Verification items for the finished model (mm, model axes). A direction names the side the tool comes from. Round coordinates to 2 decimals unless told otherwise and drop trailing zeros. Write each loop counter-clockwise with the first axis right and the second up, starting at its lowest first coordinate (ties: lowest second). Pieces come first, ordered by that corner, then holes. Notation, with made-up numbers: M 9.25,-17 L 15.25,-17 A16 ccw 15.25,-7 Z; hole C 41.5,-37.75 d7. An arc over 180 degrees is marked long. Answer in a Markdown table with one row per item. Add a question column.
1. Sectioned sample at C-C on z = -5. Record the cut outline in (x, y), plus the area to 3 significant figures.
2. Sectioned sample at D-D on x = 3. Record the cut outline in (y, z).
3. Draft check along Y on faces 1 (the flat face through (5.85, -39.7, -36.85)), 2 (the flat face through (1, -58.005, -16)), 3 (the flat face through (1, -23, -45.183)), 4 (the cylindrical face through (0.78, -37.96, -41.69)). Enter one of: pulls with the +Y half, pulls with the -Y half, needs draft (parallel to the pull), parting line crosses it, or undercut.
4. Go/stop test with flat-tipped pins: pin 1 Ø5 at (y, z) = (-36.61, 10.3) entering from +X; pin 2 Ø2.5 at (y, z) = (3.39, 10.3) entering from -X. Record where each tip stops, or that it passes through.
5. Sectioned sample at A-A on x = 9.5. Record the cut outline in (y, z), plus the area to 3 significant figures.
6. Sectioned sample at B-B on y = -43.5. Record the cut outline in (x, z).
7. Material ranges on probe 1 along X at (y, z) = (-17, -30); probe 2 along Z at (x, y) = (2.5, -43.5); probe 3 along Y at (x, z) = (0.5, 6), recorded low to high.
8. Set-up check for faces 5 (the flat face through (5.85, -45.91, -39.82)), 6 (the flat face through (5.85, -39.7, -40.78)): record each of +Z, -Z, +X, -X, +Y, -Y from which the full face is reachable in a straight line by a thin tool's end or side.
```python
from build123d import *

# Parameters (mm, degrees)
BOSS_EXTRUDE1_DEPTH           = 1.5875
SKETCH2_R                     = 1.524
CUT_EXTRUDE1_DEPTH            = 2.54
SKETCH6_W                     = 2.413
SKETCH6_H                     = 12.7
BOSS_EXTRUDE2_DEPTH           = 8.636
BOSS_EXTRUDE2_DRAFT           = 3
BOSS_EXTRUDE2_PROFILE_2_DEPTH = 8.636
BOSS_EXTRUDE2_PROFILE_2_DRAFT = 3


with BuildPart() as part:
    # Sketch1 → Boss-Extrude1 (new body)
    with BuildSketch(Plane(origin=(0, 0, 0), x_dir=(0, 0, -1), z_dir=(1, 0, 0))):
        with BuildLine():
            Line((45.182706914, 6.18069038), (-13.097593086, 6.18069038))
            Line((-13.097593086, 6.18069038), (-13.097593086, -51.36046962))
            add(Edge.make_bspline(
                [(-13.097593086, -51.36046962), (-13.097593086, -58.00510962), (-0.650340424, -58.00510962)],
                knots=[3.141592654, 3.141592654, 3.141592654, 4.71238898, 4.71238898, 4.71238898], degree=2, weights=[1, 0.707106781, 1]))
            Line((-0.650340424, -58.00510962), (32.623659576, -58.00510962))
            add(Edge.make_bspline(
                [(32.623659576, -58.00510962), (45.182706914, -58.00510962), (45.182706914, -51.36046962)],
                knots=[4.71238898, 4.71238898, 4.71238898, 6.283185307, 6.283185307, 6.283185307], degree=2, weights=[1, 0.707106781, 1]))
            Line((45.182706914, -51.36046962), (45.182706914, -39.42246962))
            Line((45.182706914, -39.42246962), (45.182706914, 6.18069038))
        make_face()
    extrude(amount=BOSS_EXTRUDE1_DEPTH)

    # Sketch2 → Cut-Extrude1 (cut)
    with BuildSketch(Plane.ZY):
        with Locations((-42.388706914, 3.38669038)):
            Circle(SKETCH2_R)
        with Locations((10.303593086, 3.38669038)):
            Circle(SKETCH2_R)
        with Locations((-42.388706914, -36.60560962)):
            Circle(SKETCH2_R)
        with Locations((10.303593086, -36.60560962)):
            Circle(SKETCH2_R)
    extrude(amount=-CUT_EXTRUDE1_DEPTH, mode=Mode.SUBTRACT)


with BuildPart() as boss_extrude2_tool:
    # Sketch6 → Boss-Extrude2 (with draft: the straight prism first)
    with BuildSketch(Plane(origin=(1.5875, 0, 0), x_dir=(0, 0, -1), z_dir=(1, 0, 0))):
        with Locations((40.801206914, -45.82580962)):
            Rectangle(SKETCH6_W, SKETCH6_H)
    extrude(amount=BOSS_EXTRUDE2_DEPTH)
    # Boss-Extrude2: the draft: its side faces are tilted about the plane it starts from
    boss_extrude2_sides = [boss_extrude2_tool.faces().sort_by_distance(p)[0] for p in [
        (5.9055, -39.47580962, -40.801206914),
        (5.9055, -45.82580962, -39.594706914),
        (5.9055, -52.17580962, -40.801206914),
        (5.9055, -45.82580962, -42.007706914),
    ]]
    draft(boss_extrude2_sides, Plane(origin=(1.5875, 0, 0), x_dir=(0, 0, -1), z_dir=(1, 0, 0)), BOSS_EXTRUDE2_DRAFT)


with BuildPart() as part_1:
    add(part.part)

    # Boss-Extrude2: add boss_extrude2_tool
    add(boss_extrude2_tool.part)


with BuildPart() as boss_extrude2_profile_2_tool:
    # Sketch6 → Boss-Extrude2 profile 2 (with draft: the straight prism first)
    with BuildSketch(Plane(origin=(1.5875, 0, 0), x_dir=(0, 0, -1), z_dir=(1, 0, 0))):
        with Locations((36.864206914, -45.82580962)):
            Rectangle(SKETCH6_W, SKETCH6_H)
    extrude(amount=BOSS_EXTRUDE2_PROFILE_2_DEPTH)
    # Boss-Extrude2 profile 2: the draft: its side faces are tilted about the plane it starts from
    boss_extrude2_profile_2_sides = [boss_extrude2_profile_2_tool.faces().sort_by_distance(p)[0] for p in [
        (5.9055, -52.17580962, -36.864206914),
        (5.9055, -45.82580962, -38.070706914),
        (5.9055, -39.47580962, -36.864206914),
        (5.9055, -45.82580962, -35.657706914),
    ]]
    draft(boss_extrude2_profile_2_sides, Plane(origin=(1.5875, 0, 0), x_dir=(0, 0, -1), z_dir=(1, 0, 0)), BOSS_EXTRUDE2_PROFILE_2_DRAFT)


with BuildPart() as part_2:
    add(part_1.part)

    # Boss-Extrude2 profile 2: add boss_extrude2_profile_2_tool
    add(boss_extrude2_profile_2_tool.part)


solid = part_2.part
```
Geometry check:
| question | item | result |
|---|---|---|
| 1 | outline | M 0,-58.01 L 1.59,-58.01 L 1.59,6.18 L 0,6.18 Z |
| 1 | area | 102 mm2 |
| 2 | outline | M -52.1,-41.93 L -39.55,-41.93 L -39.55,-39.67 L -52.1,-39.67 Z; M -52.1,-38 L -39.55,-38 L -39.55,-35.73 L -52.1,-35.73 Z |
| 3 | face 1 | pulls with the +Y half |
| 3 | face 2 | pulls with the -Y half |
| 3 | face 3 | needs draft |
| 3 | face 4 | undercut |
| 4 | pin 1 | stops at x = 1.59 |
| 4 | pin 2 | passes through |
| 5 | outline | M -51.76,-41.59 L -39.89,-41.59 L -39.89,-40.01 L -51.76,-40.01 Z; M -51.76,-37.66 L -39.89,-37.66 L -39.89,-36.07 L -51.76,-36.07 Z |
| 5 | area | 37.6 mm2 |
| 6 | outline | M 0,-45.18 L 1.59,-45.18 L 1.59,-42.01 L 10.22,-41.56 L 10.22,-40.05 L 1.59,-39.59 L 1.59,-38.07 L 10.22,-37.62 L 10.22,-36.11 L 1.59,-35.66 L 1.59,13.1 L 0,13.1 Z |
| 7 | probe 1 | x = 0 to 1.59 |
| 7 | probe 2 | z = -41.96 to -39.64, -38.02 to -35.71 |
| 7 | probe 3 | y = -57.36 to 6.18 |
| 8 | face 5 | +X, +Y, -Y |
| 8 | face 6 | +Z, -Z, +X, +Y |
